Input: part model. Units: mm. Frame: model coordinates. A direction names the side the tool comes from. Coordinates: 2 decimals unless noted, no trailing zeros. Order: outer loops, then holes, each group sorted by start corner. A loop starts at its lowest first (then second) coordinate and runs counter-clockwise, first axis right, second up. Notation, with made-up numbers: M -28,86.25 L -8,86.25 A19 cw -8,105.25 Z; hole C 81,2.5 d3. An arc over 180 degrees is marked long. One line per item, written item: value.
```python
from build123d import *

# Parameters (mm, degrees)
BOSS_EXTRUDE2_DEPTH = 95
BOSS_EXTRUDE3_DEPTH = 95
CUT_EXTRUDE1_DEPTH  = 96
BOSS_EXTRUDE4_DEPTH = 20
BOSS_EXTRUDE5_DEPTH = 45
BOSS_EXTRUDE6_DEPTH = 2
SKETCH7_R           = 6.2
CUT_EXTRUDE2_DEPTH  = 163
SKETCH10_R          = 1.6
CUT_EXTRUDE4_DEPTH  = 38.899923452
SKETCH12_R          = 1.6
BOSS_EXTRUDE8_DEPTH = 2


with BuildPart() as part:
    # Sketch1 → Boss-Extrude2 (new body)
    with BuildSketch(Plane.XY):
        with BuildLine():
            Line((-20.699923452, 8.883949337), (-20.699923452, -8.982202672))
            ThreePointArc((-20.699923452, -8.982202672), (-1.749961726, -20.999088393), (17.2, -8.982202672))
            Line((17.2, -8.982202672), (17.2, 8.883949337))
            ThreePointArc((17.2, 8.883949337), (-1.749961726, 20.900835059), (-20.699923452, 8.883949337))
        make_face()
        with BuildLine():
            ThreePointArc((-18.699923452, -8.522605699), (-1.749961726, -18.999088393), (15.2, -8.522605699))
            Line((15.2, -8.522605699), (15.2, 8.424352365))
            ThreePointArc((15.2, 8.424352365), (-1.749961726, 18.900835059), (-18.699923452, 8.424352365))
            Line((-18.699923452, 8.424352365), (-18.699923452, -8.522605699))
        make_face(mode=Mode.SUBTRACT)
    extrude(amount=-BOSS_EXTRUDE2_DEPTH)

    # Sketch2 → Boss-Extrude3 (add)
    with BuildSketch(Plane.XY):
        with BuildLine():
            ThreePointArc((-14.278781058, 8.932450877), (-11.703080294, 10.091143081), (-8.912, 10.523199609))
            Line((-8.912, 10.523199609), (-8.912, 16.25))
            Line((-8.912, 16.25), (-8.912, 16.45))
            Line((-8.912, 16.45), (-8.712, 16.45))
            Line((-8.712, 16.45), (-3.6, 16.45))
            Line((-3.6, 16.45), (7.570975385, 16.45))
            ThreePointArc((7.570975385, 16.45), (-7.286500278, 18.074001934), (-18.699923452, 8.424352365))
            Line((-18.699923452, 8.424352365), (-14.278781058, 8.932450877))
        make_face()
        with BuildLine():
            Line((-8.912, -16.25), (-8.912, -10.621452943))
            ThreePointArc((-8.912, -10.621452943), (-11.703080294, -10.189396416), (-14.278781058, -9.030704211))
            Line((-14.278781058, -9.030704211), (-18.699923452, -8.522605699))
            ThreePointArc((-18.699923452, -8.522605699), (-7.286500278, -18.172255268), (7.570975385, -16.548253334))
            Line((7.570975385, -16.548253334), (-3.6, -16.548253334))
            Line((-3.6, -16.548253334), (-8.712, -16.548253334))
            Line((-8.712, -16.548253334), (-8.912, -16.548253334))
            Line((-8.912, -16.548253334), (-8.912, -16.25))
        make_face()
    extrude(amount=-BOSS_EXTRUDE3_DEPTH)

    # Sketch3 → Cut-Extrude1 (cut, through all)
    with BuildSketch(Plane.XY):
        with BuildLine():
            Line((7.570975385, -16.548253334), (0, -16.548253334))
            Line((0, -16.548253334), (0, -18.918114011))
            ThreePointArc((0, -18.918114011), (3.910891582, -18.133810498), (7.570975385, -16.548253334))
        make_face()
        with BuildLine():
            ThreePointArc((7.570975385, 16.45), (3.141398236, 18.258676236), (-1.6, 18.900241684))
            Line((-1.6, 18.900241684), (-1.6, 16.45))
            Line((-1.6, 16.45), (7.570975385, 16.45))
        make_face()
    extrude(amount=-CUT_EXTRUDE1_DEPTH, mode=Mode.SUBTRACT)

    # Sketch4 → Boss-Extrude4 (add)
    with BuildSketch(Plane.XY):
        with BuildLine():
            Line((-20.699923452, 8.883949337), (-20.699923452, -8.982202672))
            ThreePointArc((-20.699923452, -8.982202672), (-1.749961726, -20.999088393), (17.2, -8.982202672))
            Line((17.2, -8.982202672), (17.2, 8.883949337))
            ThreePointArc((17.2, 8.883949337), (-1.749961726, 20.900835059), (-20.699923452, 8.883949337))
        make_face()
        with BuildLine():
            Line((-18.699923452, -8.522605699), (-14.278781058, -9.030704211))
            ThreePointArc((-14.278781058, -9.030704211), (-11.703080294, -10.189396416), (-8.912, -10.621452943))
            Line((-8.912, -10.621452943), (-8.912, -16.548253334))
            Line((-8.912, -16.548253334), (0, -16.548253334))
            Line((0, -16.548253334), (0, -18.918114011))
            ThreePointArc((0, -18.918114011), (8.947628308, -15.690821488), (15.2, -8.522605699))
            Line((15.2, -8.522605699), (15.2, 8.424352365))
            ThreePointArc((15.2, 8.424352365), (8.276897691, 16.030771953), (-1.6, 18.900241684))
            Line((-1.6, 18.900241684), (-1.6, 16.45))
            Line((-1.6, 16.45), (-8.912, 16.45))
            Line((-8.912, 16.45), (-8.912, 10.523199609))
            ThreePointArc((-8.912, 10.523199609), (-11.703080294, 10.091143081), (-14.278781058, 8.932450877))
            Line((-14.278781058, 8.932450877), (-18.699923452, 8.424352365))
            Line((-18.699923452, 8.424352365), (-18.699923452, -8.522605699))
        make_face(mode=Mode.SUBTRACT)
    extrude(amount=BOSS_EXTRUDE4_DEPTH)

    # Sketch5 → Boss-Extrude5 (add)
    with BuildSketch(Plane(origin=(0, 0, -95), x_dir=(-1, 0, 0), z_dir=(0, 0, -1))):
        with BuildLine():
            Line((20.699923452, -8.982202672), (20.699923452, 8.883949337))
            ThreePointArc((20.699923452, 8.883949337), (1.749961726, 20.900835059), (-17.2, 8.883949337))
            Line((-17.2, 8.883949337), (-17.2, -8.982202672))
            ThreePointArc((-17.2, -8.982202672), (1.749961726, -20.999088393), (20.699923452, -8.982202672))
        make_face()
        with BuildLine():
            Line((-15.2, 8.424352365), (-15.2, -8.522605699))
            ThreePointArc((-15.2, -8.522605699), (-8.947628308, -15.690821488), (0, -18.918114011))
            Line((0, -18.918114011), (0, -16.548253334))
            Line((0, -16.548253334), (8.912, -16.548253334))
            Line((8.912, -16.548253334), (8.912, -10.621452943))
            ThreePointArc((8.912, -10.621452943), (11.703080294, -10.189396416), (14.278781058, -9.030704211))
            Line((14.278781058, -9.030704211), (18.699923452, -8.522605699))
            Line((18.699923452, -8.522605699), (18.699923452, 8.424352365))
            Line((18.699923452, 8.424352365), (14.278781058, 8.932450877))
            ThreePointArc((14.278781058, 8.932450877), (11.703080294, 10.091143081), (8.912, 10.523199609))
            Line((8.912, 10.523199609), (8.912, 16.45))
            Line((8.912, 16.45), (1.6, 16.45))
            Line((1.6, 16.45), (1.6, 18.900241684))
            ThreePointArc((1.6, 18.900241684), (-8.276897691, 16.030771953), (-15.2, 8.424352365))
        make_face(mode=Mode.SUBTRACT)
    extrude(amount=BOSS_EXTRUDE5_DEPTH)

    # Sketch6 → Boss-Extrude6 (add)
    with BuildSketch(Plane(origin=(0, 0, -140), x_dir=(-1, 0, 0), z_dir=(0, 0, -1))):
        with BuildLine():
            Line((20.699923452, -8.982202672), (20.699923452, 8.883949337))
            ThreePointArc((20.699923452, 8.883949337), (1.749961726, 20.900835059), (-17.2, 8.883949337))
            Line((-17.2, 8.883949337), (-17.2, -8.982202672))
            ThreePointArc((-17.2, -8.982202672), (1.749961726, -20.999088393), (20.699923452, -8.982202672))
        make_face()
    extrude(amount=BOSS_EXTRUDE6_DEPTH)

    # Sketch7 → Cut-Extrude2 (cut, through all)
    with BuildSketch(Plane(origin=(0, 0, -142), x_dir=(-1, 0, 0), z_dir=(0, 0, -1))):
        with BuildLine():
            ThreePointArc((0.364575498, 16.400766737), (-4.6, 10.3251), (0.364575498, 4.249433263))
            Line((0.364575498, 4.249433263), (0.364575498, 16.400766737))
        make_face()
        with BuildLine():
            Line((0.364575498, 16.400766737), (0.364575498, 4.249433263))
            ThreePointArc((0.364575498, 4.249433263), (5.523032506, 5.524077613), (7.8, 10.3251))
            ThreePointArc((7.8, 10.3251), (5.523032506, 15.126122387), (0.364575498, 16.400766737))
        make_face()
        with Locations((1.6, -8.707225505)):
            Circle(SKETCH7_R)
    extrude(amount=-CUT_EXTRUDE2_DEPTH, mode=Mode.SUBTRACT)

    # Sketch10 → Cut-Extrude4 (cut, through all)
    with BuildSketch(Plane(origin=(17.2, 0, 0), x_dir=(0, 0, -1), z_dir=(1, 0, 0))):
        with Locations((91.5, -0.049126667)):
            Circle(SKETCH10_R)
        with Locations((3.5, -0.049126667)):
            Circle(SKETCH10_R)
        with Locations((-5.375, -0.049126667)):
            Circle(SKETCH10_R)
        with Locations((-15.125, -0.024563334)):
            Circle(SKETCH10_R)
    extrude(amount=-CUT_EXTRUDE4_DEPTH, mode=Mode.SUBTRACT)

    # Sketch12 → Boss-Extrude8 (add)
    with BuildSketch(Plane.ZY.offset(20.699923452)):
        with Locations((-91.5, -0.049126667)):
            Circle(SKETCH12_R)
        with Locations((-3.5, -0.049126667)):
            Circle(SKETCH12_R)
    extrude(amount=-BOSS_EXTRUDE8_DEPTH)


solid = part.part
```
(1) Ray query, line 1 (Y direction, x = -1.6, z = -140.85); line 2 (X direction, y = -3, z = -94); line 3 (Y direction, x = -1, z = -38). Return the intervals inside material, ascending. Write a range as from..to.
Data:
line 1: y = -21..-14.91, -2.51..4.13, 16.53..20.9
line 2: x = -20.7..-18.7, 15.2..17.2
line 3: y = -20.99..-16.55, 18.89..20.89
(2) Draft query along Y for faces 1 (the cylindrical face through (-1.418, -20.996, -59.866)), 2 (the cylindrical face through (16.214, 0.046, 16.723)), 3 (the flat face through (17.2, 0, -60)). Return one class per face: released by +Y, released by -Y, zero draft, split by the parting line, or undercut.
Data:
face 1: released by -Y
face 2: undercut
face 3: zero draft
(3) Cut plane B-B on x = 9.5. Output: boundary loops of the cut face in (y, z), plus the area to 3 significant figures.
Data:
outline: M -17.72,-142 L 17.62,-142 L 17.62,20 L 15.2,20 L 15.2,-140 L -15.3,-140 L -15.3,20 L -17.72,20 Z
area: 846 mm2
(4) First-contact query: pin 1 (2.5 mm diameter, centred on y = 18, z = -44.5, fed in from +X); pin 2 (6 mm diameter, centred on y = -9.5, z = -99.5, fed in from +X); pin 3 (3 mm diameter, centred on x = -12, z = -61, fed in from +Y); pin 4 (5 mm diameter, centred on x = -7.5, z = -40.5, fed in from -Y). Flat tips, straight axial feed; report the tip coordinate or a pass-through.
Data:
pin 1: stops at x = 10.77
pin 2: stops at x = 17.2
pin 3: stops at y = 18.99
pin 4: stops at y = -20.75
(5) Cut plane A-A on z = -25. Output: boundary loops of the cut face in (x, y), plus the area to 3 significant figures.
Data:
outline: M -20.7,-8.98 A20.95 ccw 17.2,-8.98 L 17.2,8.88 A20.95 ccw -20.7,8.88 Z; hole M -18.7,-8.52 L -14.28,-9.03 A10.53 ccw -8.91,-10.62 L -8.91,-16.55 L 0,-16.55 L 0,-18.92 A18.95 ccw 15.2,-8.52 L 15.2,8.42 A18.95 ccw -1.6,18.9 L -1.6,16.53 A6.2 ccw -2.56,16.45 L -8.91,16.45 L -8.91,10.52 A10.53 ccw -14.28,8.93 L -18.7,8.42 Z
area: 373 mm2
(6) Access query for faces 4 (the cylindrical face through (-11.67, -10.2, -58.88)), 5 (the cylindrical face through (16.214, 0.021, 6.973)). Directions: +Z, -Z, +X, -X, +Y, -Y. A direction counts if a zero-diameter tool reaches every point of the face in a straight line with its end or side. Return the directions, or none.
Data:
face 4: +Z
face 5: +X, -X
(7) Cut plane C-C on z = -91.5. Output: boundary loops of the cut face in (x, y), plus the area to 3 significant figures.
Data:
outline: M -20.7,-8.98 A20.95 ccw 17.2,-8.98 L 17.2,-1.65 L 15.2,-1.65 L 15.2,-8.52 A18.95 cw 0,-18.92 L 0,-16.55 L -8.91,-16.55 L -8.91,-10.62 A10.53 cw -14.28,-9.03 L -18.7,-8.52 L -18.7,8.42 L -14.28,8.93 A10.53 cw -8.91,10.52 L -8.91,16.45 L -2.56,16.45 A6.2 cw -1.6,16.53 L -1.6,18.9 A18.95 cw 15.2,8.42 L 15.2,1.55 L 17.2,1.55 L 17.2,8.88 A20.95 ccw -20.7,8.88 Z
area: 366 mm2
